from build123d import *

# Parameters (mm, degrees)
F0_W     = 240
F0_H     = 150
F1_DEPTH = 1
F4_W     = 1
F4_H     = 150


with BuildPart() as f1:
    # F0 (on Front) → F1 (new body)
    with BuildSketch(Plane.XZ):
        with Locations((38.595604, 1.143629)):
            Rectangle(F0_W, F0_H)
    extrude(amount=F1_DEPTH)

    # F5: sweep along a path in F3
    with BuildLine(Plane(origin=(0, 0, -73.856371), x_dir=(1, 0, 0), z_dir=(0, 0, -1))) as f5_path:
        Line((-115.624746, 27.287086), (-84.538908, 2.11427))
        ThreePointArc((-84.538908, 2.11427), (-83.06134, 1.286793), (-81.392306, 1))
    # F4 (on face) → F5 (sweep)
    with BuildSketch(Plane(origin=(-81.404396, 0, 0), x_dir=(0, -1, 0), z_dir=(-1, 0, 0))):
        with Locations((0.5, 1.143629)):
            Rectangle(F4_W, F4_H)
    sweep(path=f5_path.line)


solid = f1.part
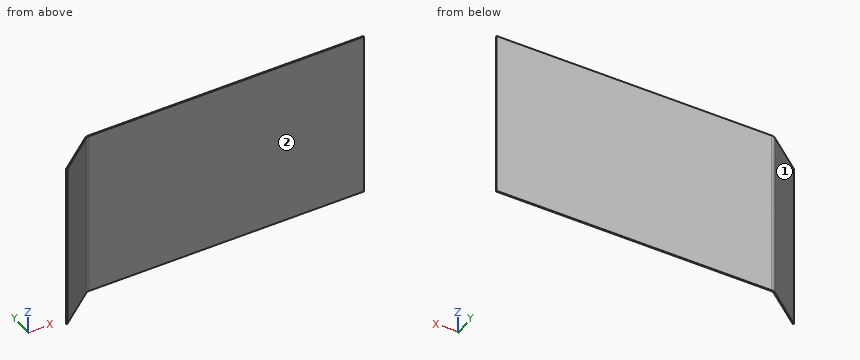
For this review, take the finished solid that the model builds, in its own axes (mm). Face numbers are marked on the shaded views. A direction names the side the tool comes from. Give positions to 0.01 mm unless a question says otherwise; leave off trailing zeros. Loops run counter-clockwise (first coordinate to the right, second up) from the corner with the lowest first, then second, coordinate; pieces in that order, holes last. Notation, with made-up numbers: (4, -28) -> (47, -28) arc R19 cw to (47, -12) -> close; hole circle Ø4 at (23.5, -34.75). An arc over 180 degrees is marked (long way). One line per question, with ' | ' between items.
1) We need section C-C (y = -5.5). Write out the cut boundary in (x, z).
Resolved:
outline: (-90.31, -73.86) -> (-88.72, -73.86) -> (-88.72, 76.14) -> (-90.31, 76.14) -> close
2) For the marked faces 1 and 2, list the 3-axis set-ups (+Z, -Z, +X, -X, +Y, -Y) from which the entire face can be reached by the end or side of a thin tool; tool diameter is ignored.
Resolved:
face 1: +Z, -Z, -X, +Y | face 2: +Z, -Z, +X, -Y
3) Insertion check: pin 1 Ø5 at (x, z) = (-60.5, -57.5) entering from -Y; pin 2 Ø10 at (y, z) = (-23, 10) entering from -X. Each pin has a flat end and moves straight along its axis. Give the tip position at first contact, or say it passes through.
Resolved:
pin 1: stops at y = -1 | pin 2: stops at x = -116.25
4) We need section B-B (x = -3). Write out the cut boundary in (y, z), plus the area to 3 significant figures.
Resolved:
outline: (-1, -73.86) -> (0, -73.86) -> (0, 76.14) -> (-1, 76.14) -> close | area: 150 mm2
5) To check wall thickness, follow probe 1 along Y at (x, z) = (-69, 21); probe 2 along Y at (x, z) = (-84.5, -62); probe 3 along X at (y, z) = (-18.25, 2). State the ranges of each line that lie inside material, in increasing order.
Resolved:
probe 1: y = -1 to 0 | probe 2: y = -2.08 to -0.87 | probe 3: x = -106.05 to -104.46
